from build123d import *

# Parameters (mm, degrees)
BOSS_EXTRUDE1_DEPTH     = 6.35
F_3_4_CLEARANCE_HOLE1_D = 19.44624
FILLET1_R               = 5
F_6_CLEARANCE_HOLE1_D   = 3.6576


with BuildPart() as part:
    # Sketch1 → Boss-Extrude1 (new body)
    with BuildSketch(Plane(origin=(0, 0, 0), x_dir=(1, 0, 0), z_dir=(0, 1, 0))):
        with BuildLine():
            Line((-17.5, -10), (-45, -10))
            Line((-45, -10), (-45, 10))
            Line((-45, 10), (45, 10))
            Line((45, 10), (45, -10))
            Line((45, -10), (17.5, -10))
            ThreePointArc((17.5, -10), (0, -27.5), (-17.5, -10))
        make_face()
    extrude(amount=BOSS_EXTRUDE1_DEPTH)

    # 3/4 Clearance Hole1 (through all)
    with Locations(Plane(origin=(0, 6.35, 0), x_dir=(1, 0, 0), z_dir=(0, 1, 0))):
        with Locations((0, -10)):
            Hole(F_3_4_CLEARANCE_HOLE1_D / 2)

    # Fillet1
    fillet1_edges = [part.edges().sort_by_distance(p)[0] for p in [
        (-45, 3.175, -10),
        (45, 3.175, -10),
        (45, 3.175, 10),
        (17.5, 3.175, 10),
        (-17.5, 3.175, 10),
        (-45, 3.175, 10),
    ]]
    fillet(fillet1_edges, radius=FILLET1_R)

    # #6 Clearance Hole1 (through all)
    with Locations(Plane(origin=(0, 6.35, 0), x_dir=(1, 0, 0), z_dir=(0, 1, 0))):
        with Locations((-35, -0.465), (35, -0.465)):
            Hole(F_6_CLEARANCE_HOLE1_D / 2)


solid = part.part
Could you check a few things on this model? Use its own coordinates, in mm. A direction names the side the tool comes from. Give positions to 0.01 mm unless a question says otherwise; leave off trailing zeros. Loops run counter-clockwise (first coordinate to the right, second up) from the corner with the lowest first, then second, coordinate; pieces in that order, holes last. Notation, with made-up numbers: M 78,54 L 126,54 A25 cw 126,82 Z; hole C 12.5,89 d1. An arc over 180 degrees is marked long. Answer as a JSON object with one key per item and string values.
Q1. If I drill on probe 1 along Z at (x, y) = (35, 3); probe 2 along Z at (x, y) = (-27, 3.75); probe 3 along X at (y, z) = (1.75, 12.5), over which ranges is the centre line in solid material (lowest first)? Write a range as [from, to].
Values found:
{"probe 1": "z = [-10, -1.36], [2.29, 10]", "probe 2": "z = [-10, 10]", "probe 3": "x = [-17.61, -9.4], [9.4, 17.61]"}
Q2. For faces 4 (the cylindrical face through (-44, 3, -8)), 5 (the flat face through (-31, 3, 10)), 6 (the flat face through (31, 3, 10)), which set-ups out of +Z, -Z, +X, -X, +Y, -Y let a thin tool reach every point of the face, with its end or its side?
Values found:
{"face 4": "-Z, -X, +Y, -Y", "face 5": "+Z, -X, +Y, -Y", "face 6": "+Z, +X, +Y, -Y"}
Q3. Suppose I cut it at D-D, the plane x = 0. List the corners of the cut face in (y, z) for me.
Values found:
{"outline": "M 0,-10 L 6.35,-10 L 6.35,0.28 L 0,0.28 Z; M 0,19.72 L 6.35,19.72 L 6.35,27.5 L 0,27.5 Z"}
Q4. If we mould it in two halves opening along X, with no side actions, what happens to faces 1 (the flat face through (-45, 3, 0)), 2 (the cylindrical face through (43, 3, -9)), 3 (the cylindrical face through (33.256, 3.131, -0.084))? For each: pulls with the +X half, pulls with the -X half, needs draft (parallel to the pull), parting line crosses it, or undercut.
Values found:
{"face 1": "pulls with the -X half", "face 2": "pulls with the +X half", "face 3": "undercut"}
Q5. Suppose I cut it at C-C, the plane y = 3.75. List the corners of the cut face in (x, z) for me (3 decimals).
Values found:
{"outline": "M -45,-5 A5 ccw -40,-10 L 40,-10 A5 ccw 45,-5 L 45,5 A5 ccw 40,10 L 21.937,10 A5 cw 17.062,13.889 A17.5 ccw -17.062,13.889 A5 cw -21.937,10 L -40,10 A5 ccw -45,5 Z; hole C -35,0.465 d3.658; hole C 0,10 d19.446; hole C 35,0.465 d3.658"}
Q6. Suppose I cut it at A-A, the plane x = -35. List the corners of the cut face in (y, z) for me, plus the area to 3 significant figures.
Values found:
{"outline": "M 0,-10 L 6.35,-10 L 6.35,-1.36 L 0,-1.36 Z; M 0,2.29 L 6.35,2.29 L 6.35,10 L 0,10 Z", "area": "104 mm²"}
Q7. Suppose I cut it at B-B, the plane z = 1.5. List the corners of the cut face in (x, y) for me, plus the area to 3 significant figures.
Values found:
{"outline": "M -45,0 L -36.51,0 L -36.51,6.35 L -45,6.35 Z; M -33.49,0 L -4.72,0 L -4.72,6.35 L -33.49,6.35 Z; M 4.72,0 L 33.49,0 L 33.49,6.35 L 4.72,6.35 Z; M 36.51,0 L 45,0 L 45,6.35 L 36.51,6.35 Z", "area": "473 mm²"}
Q8. For P1, Ø1.5, axis at y = 3, z = 14, coming from the +X side; P2, Ø2, axis at x = -30, y = 0.5, coming from the +Z side; P3, Ø1.5, axis at y = 5.5, z = 13.5, coming from the +X side, each with a flat end and sliding along its axis, tell me the tip position at first contact or that it passes through.
Values found:
{"P1": "stops at x = 17.25", "P2": "stops at z = 10", "P3": "stops at x = 17.47"}
